Autodesk Inventor part; units mm, degrees
ref_plane "YZ Plane" through (0, 0, 0) normal (1, 0, 0) x (0, 1, 0)
ref_plane "XZ Plane" through (0, 0, 0) normal (0, 1, 0) x (-1, 0, 0)
ref_plane "XY Plane" through (0, 0, 0) normal (0, 0, 1) x (1, 0, 0)
sketch "Sketch1" plane through (0, 0, 0) normal (0, 1, 0) x (-1, 0, 0)
  line L0 (0, 0) -> (-60, 0)
  line L1 (-60, 0) -> (-60, -100)
  line L2 (-60, -100) -> (0, -100)
  line L3 (0, -100) -> (0, 0)
  line L4 (-58, -5) -> (-58, -95)
  line L5 (-5, -2) -> (-5, -3)
  line L6 (-3, -5) -> (-2, -5)
  line L7 (-55, -2) -> (-55, -3)
  line L8 (-57, -5) -> (-58, -5)
  line L9 (-55, -98) -> (-55, -97)
  line L10 (-57, -95) -> (-58, -95)
  line L11 (-5, -98) -> (-5, -97)
  line L12 (-3, -95) -> (-2, -95)
  arc A0 (-5, -3) -> (-3, -5) centre (-3, -3) ccw
  arc A1 (-57, -5) -> (-55, -3) centre (-57, -3) ccw
  arc A2 (-55, -97) -> (-57, -95) centre (-57, -97) ccw
  arc A3 (-3, -95) -> (-5, -97) centre (-3, -97) ccw
  circle A4 centre (-57, -3) radius 1
  circle A5 centre (-57, -97) radius 1
  circle A6 centre (-3, -97) radius 1
  circle A7 centre (-3, -3) radius 1
  line L13 (-5, -2) -> (-55, -2)
  line L14 (-2, -95) -> (-2, -5)
  line L15 (-55, -98) -> (-5, -98)
  point P0 (-5, -5)
  point P1 (-55, -5)
  point P2 (-55, -95)
  point P3 (-5, -95)
  dimension "d0" = 60
  dimension "d1" = 100
  dimension "d6" = 3
  dimension "d7" = 3
  dimension "d8" = 3
  dimension "d9" = 3
  dimension "d10" = 3
  dimension "d11" = 3
  dimension "d12" = 2
  dimension "d13" = 3
  dimension "d14" = 2
  dimension "d15" = 2
  dimension "d16" = 2
  dimension "d17" = 2
extrude "Extrusion1" add sketch "Sketch1" along normal blind 2 contours L3 L2 L1 L0 | L8 A1 L7 L13 L5 A0 L6 L14 L12 A3 L11 L15 L9 A2 L10 L4
Here's how the part is built. I have some questions about the finished solid (model axes, mm). Coordinates: 2 decimals unless noted, no trailing zeros. Write each loop counter-clockwise with the first axis right and the second up, starting at its lowest first coordinate (ties: lowest second). Pieces come first, ordered by that corner, then holes. Notation, with made-up numbers: M 7,22.5 L 34,22.5 A19 ccw 34,51.5 Z; hole C 67,-28 d3. An arc over 180 degrees is marked long. Answer as CSV lines item,"result". Start each with the question number.
Q1. Suppose I cut it at A-A, the plane x = 3. List the corners of the cut face in (y, z) for me, then the cut area to 3 significant figures.
Q2. If we mould it in two halves opening along X, with no side actions, what happens to faces 1 (the cylindrical face through (58, 1, -3)), 2 (the cylindrical face through (3, 1, -96)), 3 (the flat face through (0, 1, -51)), 4 (the flat face through (30, 1, 0))? For each: pulls with the +X half, pulls with the -X half, needs draft (parallel to the pull), parting line crosses it, or undercut.
Q3. I need wall thicknesses on probe 1 along Z at (x, y) = (3, 1.55); probe 2 along Z at (x, y) = (56.5, 1.05). Which ranges of each line are inside material? Lowest first, please. Write a range as [from, to].
Q4. Suppose I cut it at B-B, the plane z = -97. List the corners of the cut face in (x, y) for me, then the cut area to 3 significant figures.
Entries:
1,outline,"M 0,-100 L 2,-100 L 2,-98 L 0,-98 Z; M 0,-96 L 2,-96 L 2,-4 L 0,-4 Z; M 0,-2 L 2,-2 L 2,0 L 0,0 Z"
1,area,"192 mm²"
2,face 1,"undercut"
2,face 2,"undercut"
2,face 3,"pulls with the -X half"
2,face 4,"needs draft"
3,probe 1,"z = [-100, -98], [-96, -4], [-2, 0]"
3,probe 2,"z = [-100, -97.87], [-96.13, -3.87], [-2.13, 0]"
4,outline,"M 0,0 L 2,0 L 2,2 L 0,2 Z; M 4,0 L 56,0 L 56,2 L 4,2 Z; M 58,0 L 60,0 L 60,2 L 58,2 Z"
4,area,"112 mm²"
